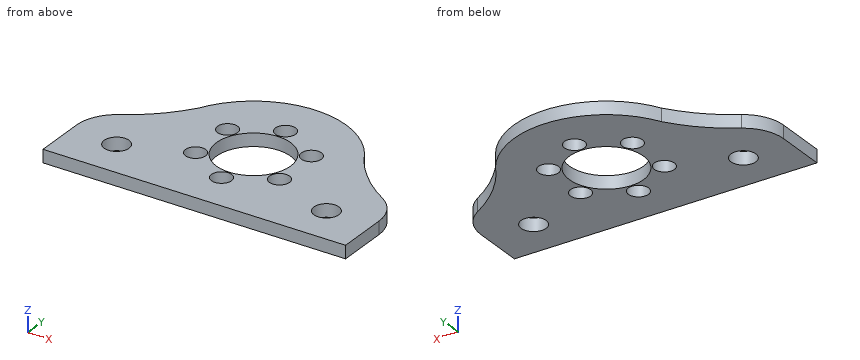
```python
from build123d import *

# Parameters (mm, degrees)
CROQUIS1_R              = 4.6
CROQUIS1_R_2            = 1.249999997
CROQUIS1_R_3            = 1.25
CROQUIS1_R_4            = 1.250000007
CROQUIS1_R_5            = 1.55
SALIENTE_EXTRUIR1_DEPTH = 1.6


with BuildPart() as part:
    # Croquis1 → Saliente-Extruir1 (new body)
    with BuildSketch(Plane.XY):
        with BuildLine():
            Line((-18.75, -11.1), (18.75, -11.1))
            Line((18.75, -11.1), (18.75, -4.852747113))
            ThreePointArc((18.75, -4.852747113), (18.116780108, -2.400965101), (16.375506293, -0.562441789))
            ThreePointArc((16.375506293, -0.562441789), (12.997975085, 1.970224072), (10.247264226, 5.172676757))
            ThreePointArc((10.247264226, 5.172676757), (0, 11.478806947), (-10.247264226, 5.172676757))
            ThreePointArc((-10.247264226, 5.172676757), (-12.997975085, 1.970224072), (-16.375506293, -0.562441789))
            ThreePointArc((-16.375506293, -0.562441789), (-18.116780108, -2.400965101), (-18.75, -4.852747113))
            Line((-18.75, -4.852747113), (-18.75, -11.1))
        make_face()
        Circle(CROQUIS1_R, mode=Mode.SUBTRACT)
        with Locations((-0.0012, 5.99880001)):
            Circle(CROQUIS1_R_2, mode=Mode.SUBTRACT)
        with Locations((5.194513192, 3.000439231)):
            Circle(CROQUIS1_R_3, mode=Mode.SUBTRACT)
        with Locations((5.195713192, -2.998360769)):
            Circle(CROQUIS1_R_3, mode=Mode.SUBTRACT)
        with Locations((0.0012, -5.9988)):
            Circle(CROQUIS1_R_3, mode=Mode.SUBTRACT)
        with Locations((-5.194513192, -3.00043923)):
            Circle(CROQUIS1_R_3, mode=Mode.SUBTRACT)
        with Locations((-5.195713248, 2.998360802)):
            Circle(CROQUIS1_R_4, mode=Mode.SUBTRACT)
        with Locations((13, -6)):
            Circle(CROQUIS1_R_5, mode=Mode.SUBTRACT)
        with Locations((-13, -6)):
            Circle(CROQUIS1_R_5, mode=Mode.SUBTRACT)
    extrude(amount=SALIENTE_EXTRUIR1_DEPTH)


solid = part.part
```
Design review of the part built by this model. Coordinates are the model's own, in mm. Give positions to 0.01 mm unless a question says otherwise; leave off trailing zeros. Write each loop counter-clockwise with the first axis right and the second up, starting at its lowest first coordinate (ties: lowest second). Pieces come first, ordered by that corner, then holes.
(1) Add section B-B (y = 0). Give the boundary of the cut face in (x, z), and give its area (3 significant figures).
Checked values:
outline: (-15.48, 0) - (-4.6, 0) - (-4.6, 1.6) - (-15.48, 1.6) - close; (4.6, 0) - (15.48, 0) - (15.48, 1.6) - (4.6, 1.6) - close
area: 34.8 mm2
(2) Add section C-C (x = -13). Give the boundary of the cut face in (y, z), and give its area (3 significant figures).
Checked values:
outline: (-11.1, 0) - (-7.55, 0) - (-7.55, 1.6) - (-11.1, 1.6) - close; (-4.45, 0) - (1.97, 0) - (1.97, 1.6) - (-4.45, 1.6) - close
area: 15.9 mm2
(3) Add section A-A (x = 0). Give the boundary of the cut face in (y, z), and give its area (3 significant figures).
Checked values:
outline: (-11.1, 0) - (-7.25, 0) - (-7.25, 1.6) - (-11.1, 1.6) - close; (-4.75, 0) - (-4.6, 0) - (-4.6, 1.6) - (-4.75, 1.6) - close; (4.6, 0) - (4.75, 0) - (4.75, 1.6) - (4.6, 1.6) - close; (7.25, 0) - (11.48, 0) - (11.48, 1.6) - (7.25, 1.6) - close
area: 13.4 mm2
(4) Add section D-D (y = -3.5). Give the boundary of the cut face in (x, z), and give its area (3 significant figures).
Checked values:
outline: (-18.57, 0) - (-6.34, 0) - (-6.34, 1.6) - (-18.57, 1.6) - close; (-4.05, 0) - (-2.98, 0) - (-2.98, 1.6) - (-4.05, 1.6) - close; (2.98, 0) - (4.05, 0) - (4.05, 1.6) - (2.98, 1.6) - close; (6.34, 0) - (18.57, 0) - (18.57, 1.6) - (6.34, 1.6) - close
area: 42.5 mm2
(5) Clearance check with flat-ended pins moving along their axes: pin 1 Ø2 at (x, y) = (5.19, 3) entering from -Z; pin 2 Ø3 at (x, y) = (-5.2, 3) entering from -Z. State where each tip first meets the part, or that it passes through.
Checked values:
pin 1: passes through
pin 2: stops at z = 0
(6) Wall thickness on line 1 along X through (y, z) = (-5.25, 0.8); line 2 along X through (y, z) = (-4, 0.6); line 3 along Y through (x, z) = (1.5, 0.3): over which ranges is each line inside the solid? List them lowest first.
Checked values:
line 1: x = -18.75 to -14.36, -11.64 to -1, 1 to 11.64, 14.36 to 18.75
line 2: x = -18.68 to -5.95, -4.44 to -2.27, 2.27 to 4.45, 5.94 to 18.68
line 3: y = -11.1 to -4.35, 4.35 to 11.38
